```python
from build123d import *

# Parameters (mm, degrees)
BOSS_EXTRUDE1_DEPTH             = 30
M3_TAPPED_HOLE1_D               = 2.5
M3_TAPPED_HOLE1_DEPTH           = 5
M3_TAPPED_HOLE1_TIP             = 0.751075774
M3_TAPPED_HOLE1_ON_FACE_2_D     = 2.5
M3_TAPPED_HOLE1_ON_FACE_2_DEPTH = 5
M3_TAPPED_HOLE1_ON_FACE_2_TIP   = 0.751075774
SKETCH7_R                       = 1.5
CUT_EXTRUDE2_DEPTH              = 5
SKETCH8_R                       = 3
CUT_EXTRUDE3_DEPTH              = 7.5
SKETCH2_R                       = 6
CUT_EXTRUDE1_DEPTH              = 12.5


with BuildPart() as part:
    # Sketch1 → Boss-Extrude1 (new body, symmetric)
    with BuildSketch(Plane.XY):
        Polygon((0, 0), (0, -2), (-2, -2), (-2, 2), (5, 2), (5, 9.5), (65, 9.5), (65, 2), (72, 2), (72, -2), (70, -2), (70, 0), (62.75, 0), (62.75, 4.5), (7.25, 4.5), (7.25, 0), align=None)
    extrude(amount=BOSS_EXTRUDE1_DEPTH, both=True)

    # M3 Tapped Hole1
    with Locations(Plane(origin=(5, 4, 17.50098961), x_dir=(0, -1, 0), z_dir=(-1, 0, 0))):
        with Locations((0, 0), (0, -38)):
            Hole(M3_TAPPED_HOLE1_D / 2, depth=M3_TAPPED_HOLE1_DEPTH)
            with Locations((0, 0, -(M3_TAPPED_HOLE1_DEPTH + M3_TAPPED_HOLE1_TIP / 2))):  # 118° drill point
                Cone(0, M3_TAPPED_HOLE1_D / 2, M3_TAPPED_HOLE1_TIP, mode=Mode.SUBTRACT)

    # M3 Tapped Hole1 on face 2
    with Locations(Plane(origin=(65, 4, 17.50098961), x_dir=(0, 0, 1), z_dir=(1, 0, 0))):
        with Locations((0, 0), (-38, 0)):
            Hole(M3_TAPPED_HOLE1_ON_FACE_2_D / 2, depth=M3_TAPPED_HOLE1_ON_FACE_2_DEPTH)
            with Locations((0, 0, -(M3_TAPPED_HOLE1_ON_FACE_2_DEPTH + M3_TAPPED_HOLE1_ON_FACE_2_TIP / 2))):  # 118° drill point
                Cone(0, M3_TAPPED_HOLE1_ON_FACE_2_D / 2, M3_TAPPED_HOLE1_ON_FACE_2_TIP, mode=Mode.SUBTRACT)

    # Sketch7 → Cut-Extrude2 (cut, through all)
    with BuildSketch(Plane(origin=(0, 2, 0), x_dir=(1, 0, 0), z_dir=(0, 1, 0))):
        with Locations((3.5, 14)):
            Circle(SKETCH7_R)
        with Locations((66.5, 14)):
            Circle(SKETCH7_R)
        with Locations((3.5, -12)):
            Circle(SKETCH7_R)
        with Locations((66.5, -12)):
            Circle(SKETCH7_R)
    extrude(amount=-CUT_EXTRUDE2_DEPTH, mode=Mode.SUBTRACT)

    # Sketch8 → Cut-Extrude3 (cut)
    with BuildSketch(Plane(origin=(0, 9.5, 0), x_dir=(1, 0, 0), z_dir=(0, 1, 0))):
        with Locations((3.5, 14)):
            Circle(SKETCH8_R)
        with Locations((3.5, -12)):
            Circle(SKETCH8_R)
        with Locations((66.5, 14)):
            Circle(SKETCH8_R)
        with Locations((66.5, -12)):
            Circle(SKETCH8_R)
    extrude(amount=-CUT_EXTRUDE3_DEPTH, mode=Mode.SUBTRACT)

    # Sketch2 → Cut-Extrude1 (cut, through all)
    with BuildSketch(Plane(origin=(0, 9.5, 0), x_dir=(1, 0, 0), z_dir=(0, 1, 0))):
        with Locations((15, 16)):
            Circle(SKETCH2_R)
        with Locations((55, 16)):
            Circle(SKETCH2_R)
        with Locations((15, -14)):
            Circle(SKETCH2_R)
        with Locations((55, -14)):
            Circle(SKETCH2_R)
    extrude(amount=-CUT_EXTRUDE1_DEPTH, mode=Mode.SUBTRACT)


solid = part.part
```
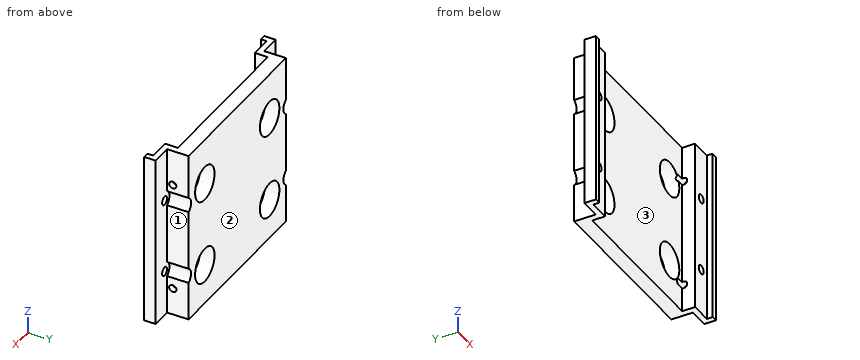
Check sheet for the modelled part. Datum: model origin and axes. Units: mm. Face numbers are marked on the shaded views. Round coordinates to 2 decimals unless told otherwise and drop trailing zeros. Write each loop counter-clockwise with the first axis right and the second up, starting at its lowest first coordinate (ties: lowest second). Pieces come first, ordered by that corner, then holes. Notation, with made-up numbers: (-40, 89) -> (-20, 89) arc R15 cw to (-20, 95) -> close; hole circle Ø5 at (11.5, 4.5). An arc over 180 degrees is marked (long way). Put each result on its own line as item: value.
(1) Material ranges on line 1 (Z direction, x = 66.5, y = 1.1); line 2 (X direction, y = 7.75, z = 15.5); line 3 (X direction, y = 0.8, z = 12), recorded low to high.
Values found:
line 1: z = -30 to -15.5, -12.5 to 10.5, 13.5 to 30
line 2: x = 5 to 9.19, 20.81 to 49.19, 60.81 to 65
line 3: x = -2 to 2, 5 to 7.25, 62.75 to 65, 68 to 72
(2) Go/stop test with flat-tipped pins: pin 1 Ø8 at (x, z) = (33, 16) entering from -Y; pin 2 Ø2.5 at (x, z) = (1, -14.5) entering from +Y; pin 3 Ø2.5 at (x, z) = (3.5, 12) entering from -Y; pin 4 Ø1.5 at (y, z) = (4, 17.5) entering from +X. Record where each tip stops, or that it passes through.
Values found:
pin 1: stops at y = 4.5
pin 2: stops at y = 2
pin 3: passes through
pin 4: stops at x = 59.7
(3) Sectioned sample at D-D (x = 3.5). Enter the section's corners in (y, z), plus the area to 3 significant figures.
Values found:
outline: (0, -30) -> (2, -30) -> (2, -15.5) -> (0, -15.5) -> close; (0, -12.5) -> (2, -12.5) -> (2, 10.5) -> (0, 10.5) -> close; (0, 13.5) -> (2, 13.5) -> (2, 30) -> (0, 30) -> close
area: 108 mm^2
(4) Sectioned sample at A-A (x = 55). Enter the section's corners in (y, z).
Values found:
outline: (4.5, -30) -> (9.5, -30) -> (9.5, -22) -> (4.5, -22) -> close; (4.5, -10) -> (9.5, -10) -> (9.5, 8) -> (4.5, 8) -> close; (4.5, 20) -> (9.5, 20) -> (9.5, 30) -> (4.5, 30) -> close
(5) Sectioned sample at B-B (z = 12). Count the separate pieces of the cut face and the enclosed holes in it, plus the area to 3 significant figures.
Values found:
separate pieces: 5
enclosed holes: 0
area: 209 mm^2
(6) Sectioned sample at C-C (z = -5). Enter the section's corners in (x, y).
Values found:
outline: (-2, -2) -> (0, -2) -> (0, 0) -> (7.25, 0) -> (7.25, 4.5) -> (62.75, 4.5) -> (62.75, 0) -> (70, 0) -> (70, -2) -> (72, -2) -> (72, 2) -> (65, 2) -> (65, 9.5) -> (5, 9.5) -> (5, 2) -> (-2, 2) -> close
(7) Mould release check, pull along X, two halves, no side actions. Record for the marked faces 1, 2 and 3: released by +X, released by -X, zero draft, split by the parting line, or undercut.
Values found:
face 1: released by +X
face 2: zero draft
face 3: undercut
